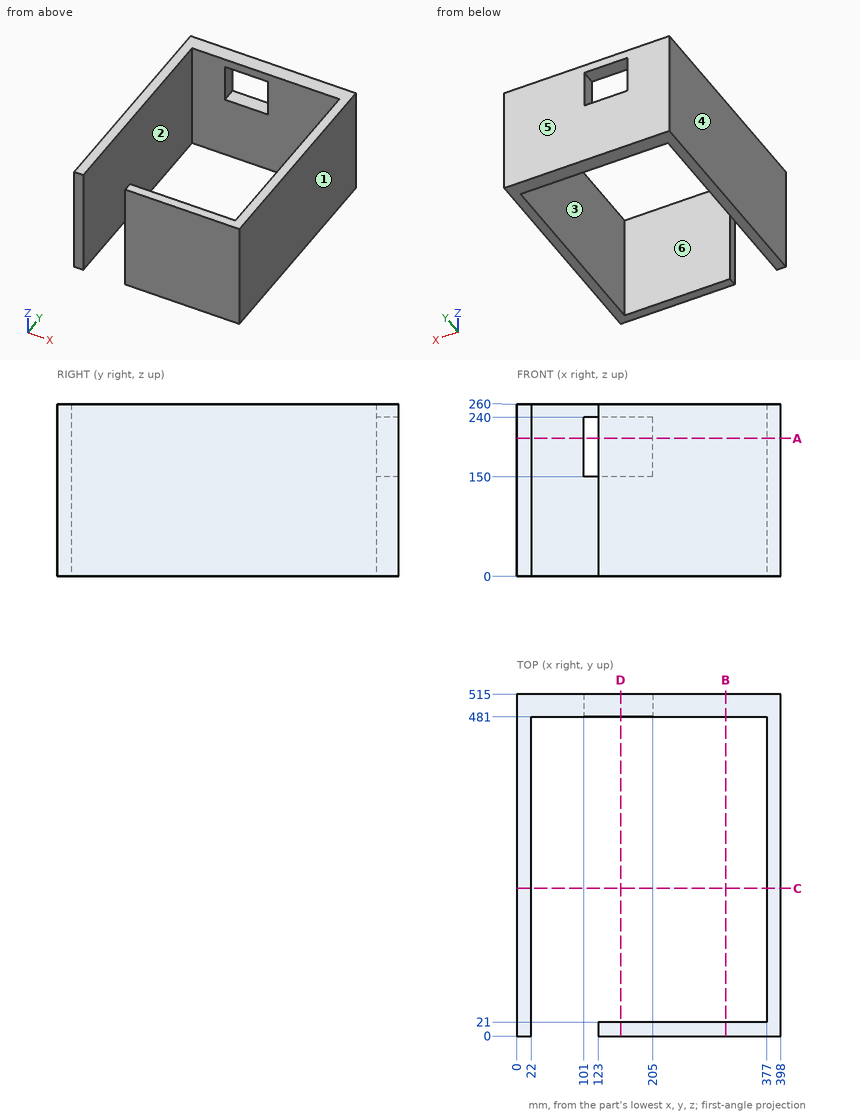
Verification items for this drawing (mm, ordinates from the low corner). A direction names the side the tool comes from. Round coordinates to 2 decimals unless told otherwise and drop trailing zeros. Order: outer loops, then holes, each group sorted by start corner. A loop starts at its lowest first (then second) coordinate and runs counter-clockwise, first axis right, second up. Notation, with made-up numbers: M 83.25,58.5 L 140.25,58.5 A23 ccw 140.25,78.5 Z; hole C 20.25,-31.5 d2. An arc over 180 degrees is marked long. Answer in a Markdown table with one row per item. Add a question column.
Item 1: Material ranges on L1, parallel to Y at x = 286, z = 70.5; L2, parallel to X at y = 184, z = 82; L3, parallel to X at y = 493, z = 182.5, recorded low to high. Write a range as [from, to].
Item 2: Sectioned sample at D-D, the plane x = 156.5. Enter the section's corners in (y, z), plus the area to 3 significant figures.
Item 3: Set-up check for the marked faces 1, 2 and 3: record each of +Z, -Z, +X, -X, +Y, -Y from which the full face is reachable in a straight line by a thin tool's end or side.
Item 4: Sectioned sample at B-B, the plane x = 315. Enter the section's corners in (y, z).
Item 5: Draft check along Y on the marked faces 4, 5 and 6. Enter one of: released by +Y, released by -Y, zero draft, split by the parting line, or undercut.
Item 6: Sectioned sample at A-A, the plane z = 208. Enter the section's corners in (x, y), plus the area to 3 significant figures.
Item 7: Sectioned sample at C-C, the plane y = 222.5. Enter the section's corners in (x, z).
Filled in:
| question | item | result |
|---|---|---|
| 1 | L1 | y = [0, 21], [481, 515] |
| 1 | L2 | x = [0, 22], [377, 398] |
| 1 | L3 | x = [0, 101], [205, 398] |
| 2 | outline | M 0,0 L 21,0 L 21,260 L 0,260 Z; M 481,0 L 515,0 L 515,150 L 481,150 Z; M 481,240 L 515,240 L 515,260 L 481,260 Z |
| 2 | area | 11,200 mm² |
| 3 | face 1 | +Z, -Z, +X, +Y, -Y |
| 3 | face 2 | +Z, -Z, -Y |
| 3 | face 3 | +Z, -Z |
| 4 | outline | M 0,0 L 21,0 L 21,260 L 0,260 Z; M 481,0 L 515,0 L 515,260 L 481,260 Z |
| 5 | face 4 | zero draft |
| 5 | face 5 | released by +Y |
| 5 | face 6 | undercut |
| 6 | outline | M 0,0 L 22,0 L 22,481 L 101,481 L 101,515 L 0,515 Z; M 123,0 L 398,0 L 398,515 L 205,515 L 205,481 L 377,481 L 377,21 L 123,21 Z |
| 6 | area | 36,000 mm² |
| 7 | outline | M 0,0 L 22,0 L 22,260 L 0,260 Z; M 377,0 L 398,0 L 398,260 L 377,260 Z |
